Autodesk Inventor part; units mm, degrees
ref_plane "YZ Plane" through (0, 0, 0) normal (1, 0, 0) x (0, 1, 0)
ref_plane "XZ Plane" through (0, 0, 0) normal (0, 1, 0) x (-1, 0, 0)
ref_plane "XY Plane" through (0, 0, 0) normal (0, 0, 1) x (1, 0, 0)
sketch "Sketch1" plane through (0, 0, 0) normal (0, 0, 1) x (1, 0, 0)
  line L0 (25, -5) -> (-25, -5)
  line L1 (-25, -5) -> (-25, 5)
  line L2 (-25, 5) -> (25, 5)
  line L3 (25, -5) -> (-25, 5) construction
  line L4 (-25, -5) -> (25, 5) construction
  line L5 (25, -5) -> (35, -5)
  line L6 (35, -5) -> (35, 35)
  line L7 (25, 35) -> (25, 5)
  line L8 (25, 35) -> (-265, 35)
  line L9 (-265, 35) -> (-265, 50)
  line L10 (-265, 50) -> (35, 50)
  line L11 (35, 50) -> (35, 35)
  point P0 (0, 0)
  dimension "d0" = 50
  dimension "d1" = 10
  dimension "d2" = 10
  dimension "d3" = 40
  dimension "d4" = 300
  dimension "d5" = 15
extrude "Extrusion1" add sketch "Sketch1" along normal mid plane 90
sketch "Sketch4" plane through (-25, -5, 45) normal (0, -1, 0) x (1, 0, 0)
  circle A0 centre (25, -45) radius 1
  dimension "d17" = 2
extrude "Extrusion4" cut sketch "Sketch4" against normal through all
sketch "Sketch5" plane through (-265, 35, 45) normal (-1, 0, 0) x (0, 0, 1)
  line L0 (-7.5, 7) -> (-82.5, 7)
  line L1 (-82.5, 7) -> (-82.5, 2)
  line L2 (-7.5, 2) -> (-7.5, 7)
  line L3 (-7.5, 7) -> (-82.5, 2) construction
  line L4 (-82.5, 7) -> (-7.5, 2) construction
  line L5 (-72.5, 2) -> (-72.5, 0)
  line L6 (-72.5, 0) -> (-17.5, 0)
  line L7 (-17.5, 0) -> (-17.5, 2)
  line L8 (-82.5, 2) -> (-72.5, 2)
  line L9 (-17.5, 2) -> (-7.5, 2)
  point P0 (-45, -35)
  point P1 (-45, 4.5)
  dimension "d32" = 75
  dimension "d33" = 5
  dimension "d34" = 55
sketch "Sketch6" plane through (-265, 35, 45) normal (-1, 0, 0) x (0, 0, 1)
  line L0 (-90, 15) -> (0, 15)
  line L1 (0, 15) -> (-90, 15)
  line L2 (-90, 15) -> (-90, 12.5)
  line L3 (-90, 12.5) -> (0, 12.5)
  line L4 (0, 12.5) -> (0, 15)
  point P0 (-45, -35)
  dimension "d25" = 90
  dimension "d26" = 2.5
extrude "Extrusion6" cut sketch "Sketch6" against normal blind 300
sketch "Sketch7" plane through (-265, 47.5, 45) normal (0, 1, 0) x (1, 0, 0)
  circle A0 centre (3, 45) radius 1.5
  point P0 (265, 45)
  dimension "d29" = 3
extrude "Extrusion7" cut sketch "Sketch7" against normal blind 60
extrude "Extrusion8" cut sketch "Sketch5" against normal blind 250
properties part number "kamera_feste"
Model file for the job. Use its own axes, mm. A direction names the side the tool comes from. Give positions to 0.01 mm unless a question says otherwise; leave off trailing zeros. Order: outer loops, then holes, each group sorted by start corner. A loop starts at its lowest first (then second) coordinate and runs counter-clockwise, first axis right, second up. Notation, with made-up numbers: (76.5, 46) - (134.5, 46) arc R21 cw to (134.5, 83) - close; hole circle Ø8 at (-19.75, 23). An arc over 180 degrees is marked (long way). Return JSON: item names as keys, results as strings.
1) Flat gauge pins, fed straight in: P1, Ø9, axis at y = 25.5, z = -10.5, coming from the -X side; P2, Ø2, axis at y = 38.5, z = 15.5, coming from the -X side; P3, Ø1.2, axis at x = 0, z = 0, coming from the -Y side (3 decimals); P4, Ø1.5, axis at x = -233, z = -33, coming from the -Y side. Where does each tip first touch, or does it go through?
Geometry says:
{"P1": "x = 25", "P2": "x = -15", "P3": "through", "P4": "y = 35"}
2) Cut at B-B, the plane z = 32.5. Give the cut face in (x, y).
Geometry says:
{"outline": "(-265, 35) - (25, 35) - (25, 5) - (-25, 5) - (-25, -5) - (35, -5) - (35, 47.5) - (-265, 47.5) - (-265, 42) - (-15, 42) - (-15, 37) - (-265, 37) - close"}
3) Cut at C-C, the plane y = 18.5. Give the cut face in (x, z).
Geometry says:
{"outline": "(25, -45) - (35, -45) - (35, 45) - (25, 45) - close"}
4) Probe line 1 (Z direction, x = -262, y = 44); line 2 (Y direction, x = -9.5, z = -34.5); line 3 (Z direction, x = 0, y = 43). List the from-to ranges inside material, lowest first. Write a range as from..to.
Geometry says:
{"line 1": "-45..-1.5, 1.5..45", "line 2": "-5..5, 35..47.5", "line 3": "-45..-1, 1..45"}
5) 3-axis set-ups, long thin cutter, end or side, ignore diameter. For faces 4 (the flat face through (-25, 0, -1)), 5 (the flat face through (-142, 42, 1)), 6 (the flat face through (25, 20, -1)): which of +Z, -Z, +X, -X, +Y, -Y reach the whole face in a straight line?
Geometry says:
{"face 4": "+Z, -Z, -X, -Y", "face 5": "-X", "face 6": "+Z, -Z, -X"}
6) Pull direction Z, two halves, no side cores. Call faces 1 (the flat face through (-142, 40, -37.5)), 2 (the flat face through (-93, 37, -45)), 3 (the flat face through (-118, 35, -31)): pulls with the +Z half, pulls with the -Z half, needs draft (parallel to the pull), parting line crosses it, or undercut.
Geometry says:
{"face 1": "undercut", "face 2": "pulls with the -Z half", "face 3": "needs draft"}
7) Cut at D-D, the plane z = -6.5. Give the cut face in (x, y).
Geometry says:
{"outline": "(-265, 42) - (-15, 42) - (-15, 35) - (25, 35) - (25, 5) - (-25, 5) - (-25, -5) - (35, -5) - (35, 47.5) - (-265, 47.5) - close"}
8) Cut at A-A, the plane x = -204. Give the cut face in (y, z).
Geometry says:
{"outline": "(35, -45) - (47.5, -45) - (47.5, 45) - (35, 45) - (35, 27.5) - (37, 27.5) - (37, 37.5) - (42, 37.5) - (42, -37.5) - (37, -37.5) - (37, -27.5) - (35, -27.5) - close"}
